Verification items for the finished model (mm, model axes). A direction names the side the tool comes from. Round coordinates to 2 decimals unless told otherwise and drop trailing zeros. Order: outer loops, then holes, each group sorted by start corner. A loop starts at its lowest first (then second) coordinate and runs counter-clockwise, first axis right, second up. Notation, with made-up numbers: (18.25, 68) -> (63.25, 68) arc R15 ccw to (63.25, 88) -> close; hole circle Ø8 at (28.5, -36). An arc over 180 degrees is marked (long way). Return JSON: item names as keys, results as strings. Group by question number.
Item 1: Draft check along Z on faces 3 (the flat face through (-27, -2.5, 10)), 4 (the flat face through (0, 0, 0)), 5 (the flat face through (11.774, 1.268, 6.955)). Enter one of: pulls with the +Z half, pulls with the -Z half, needs draft (parallel to the pull), parting line crosses it, or undercut.
Item 2: Access from +Z, -Z, +X, -X, +Y, -Y to the whole of each face (thin tool, end or side, straight path). Record for faces 1 (the flat face through (-11.774, 1.268, 13.045)), 2 (the cylindrical face through (-11.517, -1.232, 9.74)).
Item 3: Sectioned sample at B-B on y = -1.6. Record the cut outline in (x, z), plus the area to 3 significant figures.
Item 4: Depth check by flat-ended pin: pin 1 Ø2 at (x, y) = (17.5, 1) entering from -Z; pin 2 Ø3.5 at (x, z) = (14, 9.5) entering from +Y; pin 3 Ø1.2 at (y, z) = (1.5, 11) entering from -X. Enter the tip coordinate at first touch or a pass-through.
Item 5: Sectioned sample at D-D on z = 16. Record the cut outline in (x, y).
Item 6: Scan lines: probe 1 along X at (y, z) = (-0.55, 10); probe 2 along X at (y, z) = (-1.75, 10); probe 3 along X at (y, z) = (-1.5, 14.5). Record each from-to range of solid material in increasing order. Write a range as from..to.
Item 7: Sectioned sample at A-A on z = 10. Record the cut outline in (x, y).
Item 8: Sectioned sample at C-C on y = 1.75. Record the cut outline in (x, z).
```python
from build123d import *

# Parameters (mm, degrees)
EXTRUDE_1_DEPTH     = 20
FILLET_1_R          = 2
SKETCH_2_R          = 2
CUT_EXTRUDE_1_DEPTH = 35.369317712
CUT_EXTRUDE_2_DEPTH = 2.5


with BuildPart() as part:
    # 草圖1 → 填料-伸長1 (new body)
    with BuildSketch(Plane.XY):
        with BuildLine():
            Line((-18.5, -2.5), (18.5, -2.5))
            ThreePointArc((18.5, -2.5), (22.25, 1.25), (26, -2.5))
            Line((26, -2.5), (27.5, -2.5))
            Line((27.5, -2.5), (27.5, 2.5))
            Line((27.5, 2.5), (-27.5, 2.5))
            Line((-27.5, 2.5), (-27.5, -2.5))
            Line((-27.5, -2.5), (-26, -2.5))
            ThreePointArc((-26, -2.5), (-22.25, 1.25), (-18.5, -2.5))
        make_face()
    extrude(amount=EXTRUDE_1_DEPTH)

    # 圓角1
    fillet_1_edges = [part.edges().sort_by_distance(p)[0] for p in [
        (-27.5, 2.5, 10),
        (27.5, 2.5, 10),
    ]]
    fillet(fillet_1_edges, radius=FILLET_1_R)

    # 草圖2 → 除料-伸長1 (cut, through all)
    with BuildSketch(Plane(origin=(0, 2.5, 0), x_dir=(1, 0, 0), z_dir=(0, 1, 0))):
        with Locations(Location((13.5, -10, 0), (0, 0, 270))):
            Circle(SKETCH_2_R)
        with Locations(Location((-13.5, -10, 0), (0, 0, 270))):
            Circle(SKETCH_2_R)
    extrude(amount=-CUT_EXTRUDE_1_DEPTH, mode=Mode.SUBTRACT)

    # 草圖3 → 除料-伸長2 (cut)
    with BuildSketch(Plane(origin=(0, 2.5, 0), x_dir=(1, 0, 0), z_dir=(0, 1, 0))):
        Polygon((13.5, -5.958548116), (10, -7.979274058), (10, -12.020725942), (13.5, -14.041451884), (17, -12.020725942), (17, -7.979274058), align=None)
        Polygon((-13.5, -5.958548116), (-17, -7.979274058), (-17, -12.020725942), (-13.5, -14.041451884), (-10, -12.020725942), (-10, -7.979274058), align=None)
    extrude(amount=-CUT_EXTRUDE_2_DEPTH, mode=Mode.SUBTRACT)


solid = part.part
```
Recorded:
{
 "1": {"face 3": "needs draft", "face 4": "pulls with the -Z half", "face 5": "undercut"},
 "2": {"face 1": "+Y", "face 2": "+Y, -Y"},
 "3": {"outline": "(-27.5, 0) -> (-25.89, 0) -> (-25.89, 20) -> (-27.5, 20) -> close; (-18.61, 0) -> (18.61, 0) -> (18.61, 20) -> (-18.61, 20) -> close; (25.89, 0) -> (27.5, 0) -> (27.5, 20) -> (25.89, 20) -> close; hole circle Ø4 at (-13.5, 10); hole circle Ø4 at (13.5, 10)", "area": "784 mm²"},
 "4": {"pin 1": "z = 0", "pin 2": "y = 0", "pin 3": "x = -27.46"},
 "5": {"outline": "(-27.5, -2.5) -> (-26, -2.5) arc R3.75 cw to (-18.5, -2.5) -> (18.5, -2.5) arc R3.75 cw to (26, -2.5) -> (27.5, -2.5) -> (27.5, 0.5) arc R2 ccw to (25.5, 2.5) -> (-25.5, 2.5) arc R2 ccw to (-27.5, 0.5) -> close"},
 "6": {"probe 1": "-27.5..-25.45, -19.05..-15.5, -11.5..11.5, 15.5..19.05, 25.45..27.5", "probe 2": "-27.5..-25.92, -18.58..-15.5, -11.5..11.5, 15.5..18.58, 25.92..27.5", "probe 3": "-27.5..-25.86, -18.64..18.64, 25.86..27.5"},
 "7": {"outline": "(-27.5, -2.5) -> (-26, -2.5) arc R3.75 cw to (-18.5, -2.5) -> (-15.5, -2.5) -> (-15.5, 0) -> (-17, 0) -> (-17, 2.5) -> (-25.5, 2.5) arc R2 ccw to (-27.5, 0.5) -> close; (-11.5, -2.5) -> (11.5, -2.5) -> (11.5, 0) -> (10, 0) -> (10, 2.5) -> (-10, 2.5) -> (-10, 0) -> (-11.5, 0) -> close; (15.5, -2.5) -> (18.5, -2.5) arc R3.75 cw to (26, -2.5) -> (27.5, -2.5) -> (27.5, 0.5) arc R2 ccw to (25.5, 2.5) -> (17, 2.5) -> (17, 0) -> (15.5, 0) -> close"},
 "8": {"outline": "(-27.06, 0) -> (27.06, 0) -> (27.06, 20) -> (-27.06, 20) -> close; hole (-17, 7.98) -> (-13.5, 5.96) -> (-10, 7.98) -> (-10, 12.02) -> (-13.5, 14.04) -> (-17, 12.02) -> close; hole (10, 7.98) -> (13.5, 5.96) -> (17, 7.98) -> (17, 12.02) -> (13.5, 14.04) -> (10, 12.02) -> close"}
}
